Build history of the part. All positions in model axes, mm. Round coordinates to 2 decimals unless told otherwise and drop trailing zeros. Write each loop counter-clockwise with the first axis right and the second up, starting at its lowest first coordinate (ties: lowest second). Pieces come first, ordered by that corner, then holes. Notation, with made-up numbers: (64, 55) -> (83, 55) arc R8 ccw to (83, 67) -> close; hole circle Ø8 at (76, 49.5). An arc over 180 degrees is marked (long way). Answer in a Markdown table with one row per item.
```python
from build123d import *

# Parameters (mm, degrees)
SKETCH_1_R               = 5
EXTRUDE_1_DEPTH          = 25
CHAMFER_1_SIZE           = 1
CUT_EXTRUDE_1_DEPTH      = 26.980762114
CUT_EXTRUDE_1_DEPTH_BACK = 26.980762114
SKETCH_2_R               = 1


with BuildPart() as part:
    # 草图1 → 凸台-拉伸1 (new, symmetric)
    with BuildSketch(Plane.XY):
        Circle(SKETCH_1_R)
    extrude(amount=EXTRUDE_1_DEPTH, both=True)

    # 倒角1
    chamfer_1_edges = [part.edges().sort_by_distance(p)[0] for p in [
        (-5, 0, -25),
        (-5, 0, 25),
    ]]
    chamfer(chamfer_1_edges, length=CHAMFER_1_SIZE)

    # 草图2 → 切除-拉伸1 (cut, two sides: drawn at the far end of the back side and taken through both)
    with BuildSketch(Plane(origin=(0, 0, 0), x_dir=(1, 0, 0), z_dir=(0, 1, 0)).offset(-CUT_EXTRUDE_1_DEPTH_BACK)):
        with Locations(Location((0, 0, 0), (0, 0, 270))):
            Circle(SKETCH_2_R)
    extrude(amount=CUT_EXTRUDE_1_DEPTH + CUT_EXTRUDE_1_DEPTH_BACK, mode=Mode.SUBTRACT)


solid = part.part
```
Q1. Wall check: line 1 (Z direction, x = 0, y = 1); line 2 (X direction, y = -1, z = 0); line 3 (X direction, y = 1.25, z = 0). Give the ranges that are in metal, low to high. Write a range as [from, to].
A:
| item | result |
|---|---|
| line 1 | [-25, -1], [1, 25] |
| line 2 | [-4.9, -1], [1, 4.9] |
| line 3 | [-4.84, -1], [1, 4.84] |
Q2. Two-plate mould, pull along X, no slides. Class faces 1 (the flat face through (0, 0, 25)), 2 (the cylindrical face through (2.307, -4.436, 0.336)), 3 (the cylindrical face through (-1, 0, 0)): released by +X, released by -X, zero draft, split by the parting line, or undercut.
A:
| item | result |
|---|---|
| face 1 | zero draft |
| face 2 | split by the parting line |
| face 3 | undercut |
Q3. Saw through at A-A on x = 0. Write the cut outline in (y, z), plus the area to 3 significant figures.
A:
| item | result |
|---|---|
| outline | (-5, -24) -> (-4, -25) -> (4, -25) -> (5, -24) -> (5, -1) -> (-5, -1) -> close; (-5, 1) -> (5, 1) -> (5, 24) -> (4, 25) -> (-4, 25) -> (-5, 24) -> close |
| area | 478 mm² |
Q4. Saw through at C-C on z = 0. Write the cut outline in (x, y).
A:
| item | result |
|---|---|
| outline | (-1, -4.9) -> (-1, 4.9) arc R5 ccw to start; (1, -4.9) arc R5 ccw to (1, 4.9) -> close |
Q5. Drop flat-ended pins along their axis: P1, Ø6, axis at x = -2, z = 0.5, coming from the -Y side; P2, Ø2, axis at y = -3, z = 11.5, coming from the -X side; P3, Ø1.5, axis at x = -1.5, z = -7.5, coming from the +Y side; P4, Ø1, axis at x = -2, z = 11, coming from the +Y side. Give the stop position or say it passes through.
A:
| item | result |
|---|---|
| P1 | y = -5 |
| P2 | x = -4.58 |
| P3 | y = 4.94 |
| P4 | y = 4.77 |
Q6. Saw through at B-B on z = 17. Write the cut outline in (x, y), plus the area to 3 significant figures.
A:
| item | result |
|---|---|
| outline | circle Ø10 at (0, 0) |
| area | 78.5 mm² |
